from build123d import *

# Parameters (mm, degrees)
ESQUISSE1_R                         = 3
BOSS_EXTRU_1_DEPTH                  = 27
DIAM_TRE_DU_PER_AGE_3_0_3_1_D       = 3
DIAM_TRE_DU_PER_AGE_3_0_3_1_DEPTH   = 24.5
DIAM_TRE_DU_PER_AGE_3_0_3_1_TIP     = 0.901290929
DIAM_TRE_DU_PER_AGE_2_5_2_5_1_D     = 2.5
DIAM_TRE_DU_PER_AGE_2_5_2_5_1_DEPTH = 3
DIAM_TRE_DU_PER_AGE_2_5_2_5_1_TIP   = 0.751075774
ENL_V_START                         = -15
ESQUISSE6_W                         = 11.750178357
ESQUISSE6_H                         = 11.384595502
ESQUISSE6_R                         = 2.25
ENL_V_MAT_EXTRU_1_DEPTH             = 6
CHANFREIN1_SIZE                     = 1
CHANFREIN2_SIZE                     = 0.75


with BuildPart() as part:
    # Esquisse1 → Boss.-Extru.1 (new body)
    with BuildSketch(Plane.XY):
        Circle(ESQUISSE1_R)
    extrude(amount=BOSS_EXTRU_1_DEPTH)

    # Diamètre du perçage Ø3.0 (3)1
    with Locations(Plane.XY.offset(27)):
        with Locations((0, 0)):
            Hole(DIAM_TRE_DU_PER_AGE_3_0_3_1_D / 2, depth=DIAM_TRE_DU_PER_AGE_3_0_3_1_DEPTH)
            with Locations((0, 0, -(DIAM_TRE_DU_PER_AGE_3_0_3_1_DEPTH + DIAM_TRE_DU_PER_AGE_3_0_3_1_TIP / 2))):  # 118° drill point
                Cone(0, DIAM_TRE_DU_PER_AGE_3_0_3_1_D / 2, DIAM_TRE_DU_PER_AGE_3_0_3_1_TIP, mode=Mode.SUBTRACT)

    # Diamètre du perçage Ø2.5 (2.5)1
    with Locations(Plane(origin=(0, 0, 0), x_dir=(-1, 0, 0), z_dir=(0, 0, -1))):
        with Locations((0, 0)):
            Hole(DIAM_TRE_DU_PER_AGE_2_5_2_5_1_D / 2, depth=DIAM_TRE_DU_PER_AGE_2_5_2_5_1_DEPTH)
            with Locations((0, 0, -(DIAM_TRE_DU_PER_AGE_2_5_2_5_1_DEPTH + DIAM_TRE_DU_PER_AGE_2_5_2_5_1_TIP / 2))):  # 118° drill point
                Cone(0, DIAM_TRE_DU_PER_AGE_2_5_2_5_1_D / 2, DIAM_TRE_DU_PER_AGE_2_5_2_5_1_TIP, mode=Mode.SUBTRACT)

    # Esquisse6 → Enlèv. mat.-Extru.1 (cut)
    with BuildSketch(Plane.XY.offset(27).offset(ENL_V_START)):
        with Locations((-0.219764127, 0.428836611)):
            Rectangle(ESQUISSE6_W, ESQUISSE6_H)
        Circle(ESQUISSE6_R, mode=Mode.SUBTRACT)
    extrude(amount=-ENL_V_MAT_EXTRU_1_DEPTH, mode=Mode.SUBTRACT)

    # Chanfrein1
    chanfrein1_edges = [part.edges().sort_by_distance(p)[0] for p in [
        (-3, 0, 0),
    ]]
    chamfer(chanfrein1_edges, length=CHANFREIN1_SIZE)

    # Chanfrein2
    chanfrein2_edges = [part.edges().sort_by_distance(p)[0] for p in [
        (-2.25, 0, 6),
    ]]
    chamfer(chanfrein2_edges, length=CHANFREIN2_SIZE - 0.0001)  # a hair under: the kernel refuses the full size


solid = part.part
Check sheet for the modelled part. Datum: model origin and axes. Units: mm. A direction names the side the tool comes from. Give positions to 0.01 mm unless a question says otherwise; leave off trailing zeros. Write each loop counter-clockwise with the first axis right and the second up, starting at its lowest first coordinate (ties: lowest second). Pieces come first, ordered by that corner, then holes. Notation, with made-up numbers: (-17.5, 73.25) -> (1.5, 73.25) arc R36 cw to (1.5, 111.25) -> close; hole circle Ø11 at (5.25, -33.75). An arc over 180 degrees is marked (long way). Use one line per item in the form item = value. Start each with the question number.
1. Thickness scan on line 1 along Y through (x, z) = (0, 1.3); line 2 along Y through (x, z) = (0, 21.5). Record the ranges inside material, lowest first. Write a range as from..to.
2. Section check D-D (z = 22). Record the cut outline in (x, y).
3. Mould release check, pull along Z, two halves, no side actions. Record for faces 3 (the flat face through (1.3, -1.3, 27)), 4 (the cylindrical face through (-0.29, 2.23, 9.41)), 5 (the cylindrical face through (0.672, 1.054, 1.191)): pulls with the +Z half, pulls with the -Z half, needs draft (parallel to the pull), parting line crosses it, or undercut.
4. Access from +Z, -Z, +X, -X, +Y, -Y to the whole of each face (thin tool, end or side, straight path). Record for faces 1 (the cylindrical face through (1.5, 0.07, 14.58)), 2 (the cylindrical face through (-3, 0, 3)).
5. Section check C-C (z = 10.75). Record the cut outline in (x, y).
Conclusion:
q1.line_1 = -3..-1.25, 1.25..3
q1.line_2 = -3..-1.5, 1.5..3
q2.outline = circle Ø6 at (0, 0); hole circle Ø3 at (0, 0)
q3.face_3 = pulls with the +Z half
q3.face_4 = undercut
q3.face_5 = needs draft
q4.face_1 = +Z
q4.face_2 = +Z, -Z
q5.outline = circle Ø4.5 at (0, 0); hole circle Ø3 at (0, 0)
